```python
from build123d import *

# Parameters (mm, degrees)
SKETCH1_W           = 110
SKETCH1_H           = 140
SKETCH1_R           = 2
BOSS_EXTRUDE1_DEPTH = 5
SKETCH2_R           = 2
BOSS_EXTRUDE2_DEPTH = 5
SKETCH3_R           = 1.4732
SKETCH3_R_2         = 13
BOSS_EXTRUDE3_DEPTH = 5


with BuildPart() as part:
    # Sketch1 → Boss-Extrude1 (new body)
    with BuildSketch(Plane.XY):
        Rectangle(SKETCH1_W, SKETCH1_H)
        with Locations((-47.5, 40)):
            Circle(SKETCH1_R, mode=Mode.SUBTRACT)
        with Locations((47.5, 40)):
            Circle(SKETCH1_R, mode=Mode.SUBTRACT)
        with Locations((-47.5, 60)):
            Circle(SKETCH1_R, mode=Mode.SUBTRACT)
        with Locations((47.5, 60)):
            Circle(SKETCH1_R, mode=Mode.SUBTRACT)
    extrude(amount=BOSS_EXTRUDE1_DEPTH)

    # Sketch2 → Boss-Extrude2 (add)
    with BuildSketch(Plane.XY):
        Polygon((-26.715730122, -70), (-55, -41.715730122), (-115, -101.715728753), (-115, -203), (-75, -203), (-75, -118.28427098), align=None)
        with Locations((-95, -185.5)):
            Circle(SKETCH2_R, mode=Mode.SUBTRACT)
        with Locations((-95, -150.5)):
            Circle(SKETCH2_R, mode=Mode.SUBTRACT)
    boss_extrude2 = extrude(amount=BOSS_EXTRUDE2_DEPTH)

    # Mirror1: Boss-Extrude2 across plane
    add(boss_extrude2.mirror(Plane(origin=(0, 0, 0), x_dir=(0, 0, 1), z_dir=(1, 0, 0))))

    # Sketch3 → Boss-Extrude3 (add)
    # profile 1 of 2: a face of its own
    with BuildSketch(Plane.XY.offset(5)):
        with BuildLine():
            ThreePointArc((-55, 49.531907673), (-151.188194001, 4.063503923), (-105.126050066, -91.841779044))
            Line((-105.126050066, -91.841779044), (-55, -41.715730122))
            Line((-55, -41.715730122), (-55, 49.531907673))
        make_face()
        with Locations((-135.79276299, -59.716409454)):
            Circle(SKETCH3_R, mode=Mode.SUBTRACT)
        with Locations((-128.22970773, 26.72970773)):
            Circle(SKETCH3_R, mode=Mode.SUBTRACT)
        with BuildLine():
            ThreePointArc((-65, -23), (-67, -21), (-65, -19))
            Line((-65, -19), (-61, -19))
            ThreePointArc((-61, -19), (-59, -21), (-61, -23))
            Line((-61, -23), (-65, -23))
        make_face(mode=Mode.SUBTRACT)
        with BuildLine():
            Line((-78.5, -40.5), (-82.5, -40.5))
            ThreePointArc((-82.5, -40.5), (-84.5, -38.5), (-82.5, -36.5))
            Line((-82.5, -36.5), (-78.5, -36.5))
            ThreePointArc((-78.5, -36.5), (-76.5, -38.5), (-78.5, -40.5))
        make_face(mode=Mode.SUBTRACT)
        with BuildLine():
            ThreePointArc((-96, -19), (-94, -21), (-96, -23))
            Line((-96, -23), (-100, -23))
            ThreePointArc((-100, -23), (-102, -21), (-100, -19))
            Line((-100, -19), (-96, -19))
        make_face(mode=Mode.SUBTRACT)
        with Locations((-80.5, -21)):
            Circle(SKETCH3_R_2, mode=Mode.SUBTRACT)
        with BuildLine():
            ThreePointArc((-82.5, -5.5), (-84.5, -3.5), (-82.5, -1.5))
            Line((-82.5, -1.5), (-78.5, -1.5))
            ThreePointArc((-78.5, -1.5), (-76.5, -3.5), (-78.5, -5.5))
            Line((-78.5, -5.5), (-82.5, -5.5))
        make_face(mode=Mode.SUBTRACT)
    # profile 2 of 2: a face of its own
    with BuildSketch(Plane.XY.offset(5)):
        with BuildLine():
            ThreePointArc((105.126050066, -91.841779044), (151.188194001, 4.063503923), (55, 49.531907673))
            Line((55, 49.531907673), (55, -41.715730122))
            Line((55, -41.715730122), (105.126050066, -91.841779044))
        make_face()
        with Locations((135.79276299, -59.716409454)):
            Circle(SKETCH3_R, mode=Mode.SUBTRACT)
        with Locations((128.22970773, 26.72970773)):
            Circle(SKETCH3_R, mode=Mode.SUBTRACT)
        with BuildLine():
            ThreePointArc((82.5, -1.5), (84.5, -3.5), (82.5, -5.5))
            Line((82.5, -5.5), (78.5, -5.5))
            ThreePointArc((78.5, -5.5), (76.5, -3.5), (78.5, -1.5))
            Line((78.5, -1.5), (82.5, -1.5))
        make_face(mode=Mode.SUBTRACT)
        with BuildLine():
            ThreePointArc((65, -19), (67, -21), (65, -23))
            Line((65, -23), (61, -23))
            ThreePointArc((61, -23), (59, -21), (61, -19))
            Line((61, -19), (65, -19))
        make_face(mode=Mode.SUBTRACT)
        with BuildLine():
            ThreePointArc((82.5, -36.5), (84.5, -38.5), (82.5, -40.5))
            Line((82.5, -40.5), (78.5, -40.5))
            ThreePointArc((78.5, -40.5), (76.5, -38.5), (78.5, -36.5))
            Line((78.5, -36.5), (82.5, -36.5))
        make_face(mode=Mode.SUBTRACT)
        with Locations((80.5, -21)):
            Circle(SKETCH3_R_2, mode=Mode.SUBTRACT)
        with BuildLine():
            Line((100, -23), (96, -23))
            ThreePointArc((96, -23), (94, -21), (96, -19))
            Line((96, -19), (100, -19))
            ThreePointArc((100, -19), (102, -21), (100, -23))
        make_face(mode=Mode.SUBTRACT)
    extrude(amount=-BOSS_EXTRUDE3_DEPTH)


solid = part.part
```
Verification items for the finished model (mm, model axes). A direction names the side the tool comes from. Give positions to 0.01 mm unless a question says otherwise; leave off trailing zeros. Loops run counter-clockwise (first coordinate to the right, second up) from the corner with the lowest first, then second, coordinate; pieces in that order, holes last. Notation, with made-up numbers: M 24,15.5 L 57,15.5 A17 ccw 57,48.5 Z; hole C 71,-20.75 d5. An arc over 180 degrees is marked long. One line per question, with ' | ' between items.
Item 1: Section check A-A, the plane y = -137. Record the cut outline in (x, z).
Completed:
outline: M -115,0 L -75,0 L -75,5 L -115,5 Z; M 75,0 L 115,0 L 115,5 L 75,5 Z
Item 2: Tool access check on faces 1 (the face through (-109.994, -96.71, 2.465)), 2 (the face through (51.196, -94.48, 2.465)), 3 (the face through (67.513, -20.428, 2.535)), 4 (the face through (109.994, -96.71, 2.465)). Record the directions out of +Z, -Z, +X, -X, +Y, -Y that give a thin tool (end or side, any length) a straight path to the whole face; none if there is none.
Completed:
face 1: +Z, -Z, -X | face 2: +Z, -Z, -Y | face 3: +Z, -Z | face 4: +Z, -Z, +X
Item 3: Section check B-B, the plane y = -82.5. Record the cut outline in (x, z).
Completed:
outline: M -123.43,0 L -39.22,0 L -39.22,5 L -123.43,5 Z; M 39.22,0 L 123.43,0 L 123.43,5 L 39.22,5 Z
Item 4: Draft check along Y on faces 5 (the face through (-2, -34, 0)), 6 (the face through (-93.487, -20.428, 2.535)), 7 (the face through (-51.196, -94.48, 2.465)). Enter one of: +Y half, -Y half, draft (parallel to the pull), parting line (faces both ways), or undercut.
Completed:
face 5: draft | face 6: undercut | face 7: -Y half
Item 5: Section check D-D, the plane z = 3.35. State how many separate pieces and enclosed holes the cut face has, plus the area to 3 significant figures.
Completed:
separate pieces: 1 | enclosed holes: 22 | area: 49,100 mm^2
Item 6: Thickness scan on line 1 (X direction, y = -150.5, z = 2.95); line 2 (X direction, y = -161, z = 1.3); line 3 (X direction, y = -13.5, z = 4.3). Record the ranges inside material, lowest first. Write a range as [from, to].
Completed:
line 1: x = [-115, -97], [-93, -75], [75, 93], [97, 115] | line 2: x = [-115, -75], [75, 115] | line 3: x = [-155.12, -91.12], [-69.88, 69.88], [91.12, 155.12]
Item 7: Depth check by flat-ended pin: P1, Ø4.5, axis at x = 47.5, y = 40, coming from the -Z side; P2, Ø1.5, axis at y = -130.5, z = 3, coming from the +X side; P3, Ø1.2, axis at x = 62.5, z = 1.5, coming from the +Y side; P4, Ø3, axis at y = -85, z = 2, coming from the +X side. Enter the tip coordinate at first touch or a pass-through.
Completed:
P1: stops at z = 0 | P2: stops at x = 115 | P3: stops at y = 51.95 | P4: stops at x = 121.96
Item 8: Section check C-C, the plane x = 19. Record the cut outline in (y, z), plus the area to 3 significant figures.
Completed:
outline: M -70,0 L 70,0 L 70,5 L -70,5 Z | area: 700 mm^2
